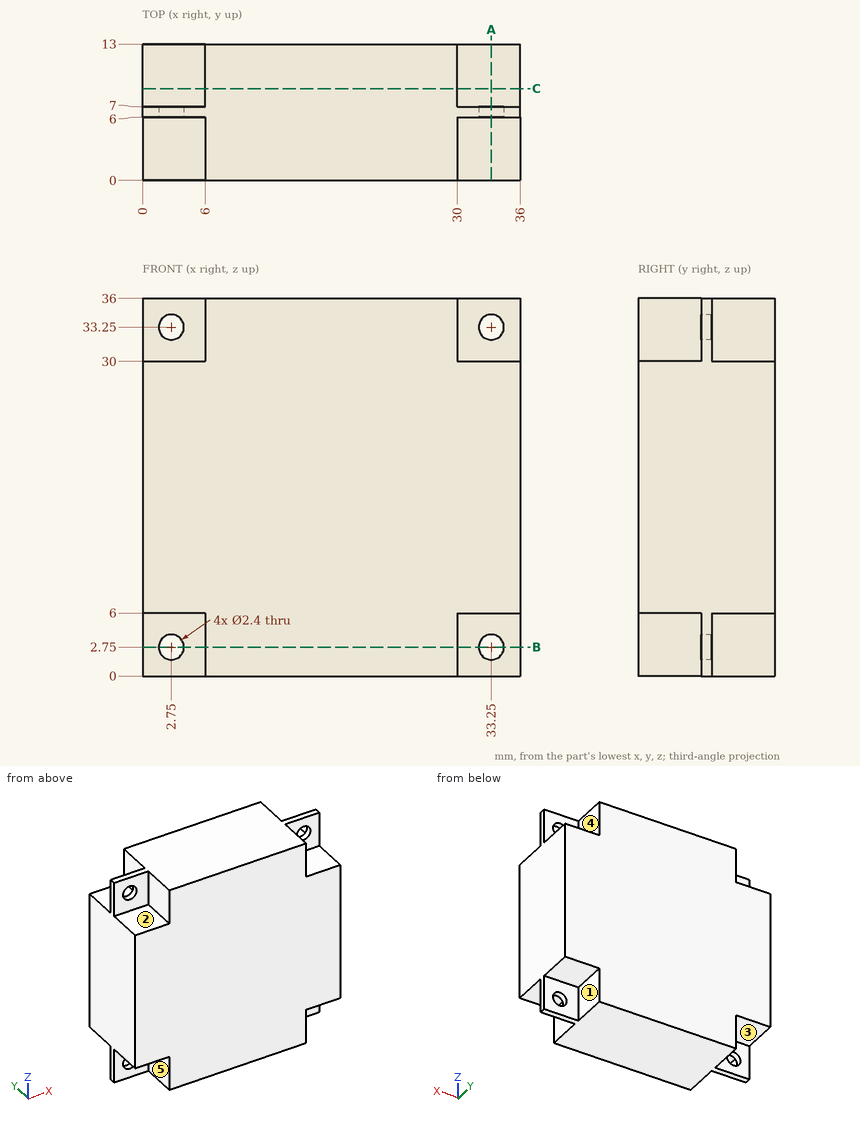
Here's the drawing with two shaded views (mm, measured from the low corner). I have some questions. A direction names the side the tool comes from. Round coordinates to 2 decimals unless told otherwise and drop trailing zeros. Loops run counter-clockwise (first coordinate to the right, second up) from the corner with the lowest first, then second, coordinate; pieces in that order, holes last.
Item 1: Suppose I cut it at C-C, the plane y = 8.75. Write out the boundary of the cut face in (x, z).
Item 2: Will these pins go through, and if not, where does the flat tip stop? pin 1 Ø1.4 at (x, z) = (2.75, 2.75) entering from +Y; pin 2 Ø10 at (x, z) = (22, 11.5) entering from -Y; pin 3 Ø5 at (y, z) = (2, 34.5) entering from -X; pin 4 Ø1.8 at (y, z) = (10.5, 2.5) entering from +X.
Item 3: Suppose I cut it at A-A, the plane x = 33.25. Write out the boundary of the cut face in (y, z).
Item 4: Please list where these lines run through material, in increasing order: L1, parallel to Z at x = 33.25, y = 6.75; L2, parallel to X at y = 1.5, z = 32.5.
Item 5: Which directions (+Z, -Z, +X, -X, +Y, -Y) give clear straight access to the entire face, cutting with the end or side of a thin tool? Please do the marked faces 1, 2, 3, 4 and 5.
Item 6: Suppose I cut it at B-B, the plane z = 2.75. Write out the boundary of the cut face in (x, y), then the cut area to 3 significant figures.
Reported:
1. outline: (0, 6) - (6, 6) - (6, 0) - (30, 0) - (30, 6) - (36, 6) - (36, 30) - (30, 30) - (30, 36) - (6, 36) - (6, 30) - (0, 30) - close
2. pin 1: passes through
2. pin 2: stops at y = 0
2. pin 3: stops at x = 6
2. pin 4: stops at x = 30
3. outline: (0, 6) - (6, 6) - (6, 3.95) - (7, 3.95) - (7, 6) - (13, 6) - (13, 30) - (7, 30) - (7, 32.05) - (6, 32.05) - (6, 30) - (0, 30) - close; (6, 0) - (7, 0) - (7, 1.55) - (6, 1.55) - close; (6, 34.45) - (7, 34.45) - (7, 36) - (6, 36) - close
4. L1: z = 0 to 1.55, 3.95 to 32.05, 34.45 to 36
4. L2: x = 6 to 30
5. face 1: -Z, +X, +Y
5. face 2: +Z, -X, -Y
5. face 3: -Z, -X, +Y
5. face 4: +Z, +X, +Y
5. face 5: -Z, -X, -Y
6. outline: (0, 6) - (1.55, 6) - (1.55, 7) - (0, 7) - close; (3.95, 6) - (6, 6) - (6, 0) - (30, 0) - (30, 6) - (32.05, 6) - (32.05, 7) - (30, 7) - (30, 13) - (6, 13) - (6, 7) - (3.95, 7) - close; (34.45, 6) - (36, 6) - (36, 7) - (34.45, 7) - close
6. area: 319 mm2
